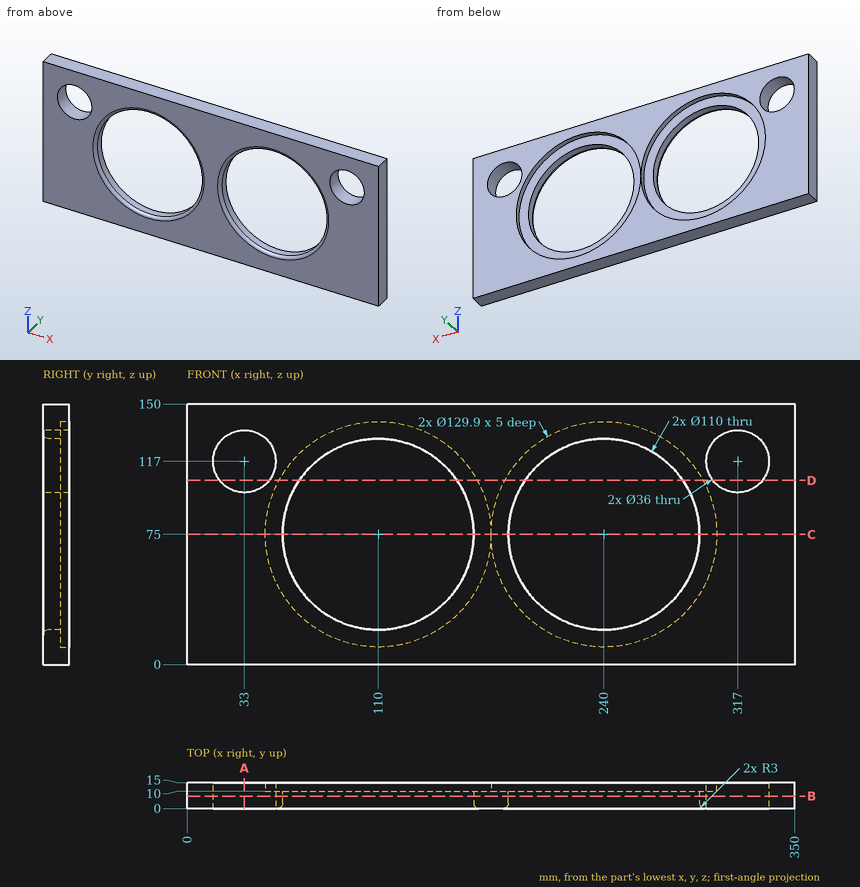
For this review, use the dimensioned drawing (mm, ordinates from the lowest corner) and the shaded views. Give positions to 0.01 mm unless a question says otherwise; leave off trailing zeros. Order: outer loops, then holes, each group sorted by start corner. A loop starts at its lowest first (then second) coordinate and runs counter-clockwise, first axis right, second up. Notation, with made-up numbers: (-0.75, 54) - (14.25, 54) arc R8 cw to (14.25, 60) - close; hole circle Ø8 at (-0.75, 46). An arc over 180 degrees is marked (long way). Write item = value, one per line. Start each with the question number.
Q1. To check wall thickness, follow L1, parallel to Z at x = 33, y = 11.75; L2, parallel to X at y = 8, z = 75; L3, parallel to Z at x = 240, y = 7.5. State the ranges of each line that lie inside material, in increasing order. Write a range as from..to.
Q2. We need section B-B on y = 7.25. State the section outline as (x, z) points.
Q3. We need section D-D on z = 106. State how many separate pieces and enclosed holes the cut face has, plus the area to 3 significant figures.
Q4. We need section C-C on z = 75. State the section outline as (x, y) points.
Q5. Clearance check with a flat-ended pin moving along its axis: pin 1 Ø1 at (x, z) = (146, 23.5) entering from +Y. State where the tip first meets the part, or that it passes through.
Q6. We need section A-A on x = 33. State the section outline as (y, z) points.
Working result:
q1.L1 = 0..99, 135..150
q1.L2 = 0..55, 165..185, 295..350
q1.L3 = 0..20, 130..150
q2.outline = (0, 0) - (350, 0) - (350, 150) - (0, 150) - close; hole circle Ø36 at (33, 117); hole circle Ø110 at (110, 75); hole circle Ø110 at (240, 75); hole circle Ø36 at (317, 117)
q3.separate_pieces = 5
q3.enclosed_holes = 0
q3.area = 1,430 mm²
q4.outline = (0, 0) - (52, 0) arc R3 ccw to (55, 3) - (55, 10) - (45.05, 10) - (45.05, 15) - (0, 15) - close; (165, 3) arc R3 ccw to (168, 0) - (182, 0) arc R3 ccw to (185, 3) - (185, 10) - (175.05, 10) - (175.05, 15) - (174.95, 15) - (174.95, 10) - (165, 10) - close; (295, 3) arc R3 ccw to (298, 0) - (350, 0) - (350, 15) - (304.95, 15) - (304.95, 10) - (295, 10) - close
q5.pin_1 = 10
q6.outline = (0, 0) - (15, 0) - (15, 99) - (0, 99) - close; (0, 135) - (15, 135) - (15, 150) - (0, 150) - close
